```python
from build123d import *

# Parameters (mm, degrees)
PAD_DEPTH = 50
FILLET_R  = 1


with BuildPart() as part:
    # Sketch → Pad (new body)
    with BuildSketch(Plane.XZ):
        Polygon((0, 0), (0, 60), (60, 60), (60, 55), (5, 55), (5, 5), (60, 5), (80, 10), (80, 5), (60, 0), align=None)
    extrude(amount=PAD_DEPTH)

    # Fillet
    fillet_edges = [part.edges().sort_by_distance(p)[0] for p in [
        (0, -25, 0),
        (60, -25, 0),
        (80, -25, 5),
        (80, -25, 10),
        (60, -25, 55),
        (60, -25, 60),
        (0, -25, 60),
        (60, -25, 5),
        (5, -25, 5),
        (5, -25, 55),
    ]]
    fillet(fillet_edges, radius=FILLET_R)


solid = part.part
```
Check sheet for the modelled part. Datum: model origin and axes. Units: mm. A direction names the side the tool comes from. Give positions to 0.01 mm unless a question says otherwise; leave off trailing zeros. Order: outer loops, then holes, each group sorted by start corner. A loop starts at its lowest first (then second) coordinate and runs counter-clockwise, first axis right, second up. Notation, with made-up numbers: M -10,26.5 L 14,26.5 A23 ccw 14,46.5 Z; hole C 74.25,89.5 d4. An arc over 180 degrees is marked long. Answer in a Markdown table with one row per item.
1) Gauge pin test, flat ends, axial feed: P1, Ø14.5, axis at y = -31, z = 25.5, coming from the +X side; P2, Ø0.9, axis at y = -27, z = 58, coming from the +X side. Record the tip position at first contact, or that the pin passes through.
Filled sheet:
| item | result |
|---|---|
| P1 | stops at x = 5 |
| P2 | stops at x = 60 |
2) Cross-section at D-D, the plane x = 67.5. Enter the section's corners in (y, z) (3 decimals).
Filled sheet:
| item | result |
|---|---|
| outline | M -50,1.875 L 0,1.875 L 0,6.875 L -50,6.875 Z |
3) Thickness scan on L1, parallel to Z at x = 15.5, y = -10; L2, parallel to X at y = -35.5, z = 58; L3, parallel to X at y = -23, z = 24. Record the ranges inside material, lowest first. Write a range as [from, to].
Filled sheet:
| item | result |
|---|---|
| L1 | z = [0, 5], [55, 60] |
| L2 | x = [0, 60] |
| L3 | x = [0, 5] |
4) Cross-section at C-C, the plane z = 18.5. Enter the section's corners in (x, y), plus the area to 3 significant figures.
Filled sheet:
| item | result |
|---|---|
| outline | M 0,-50 L 5,-50 L 5,0 L 0,0 Z |
| area | 250 mm2 |
5) Release check for a two-part mould opening along X. For faces 1 (the flat face through (33, -25, 5)), 2 (the flat face through (4.6, 0, 25.7)), 3 (the flat face through (69.815, -24.65, 2.454)) record: +X half, -X half, draft (parallel to the pull), parting line (faces both ways), or undercut.
Filled sheet:
| item | result |
|---|---|
| face 1 | undercut |
| face 2 | draft |
| face 3 | +X half |
6) Cross-section at B-B, the plane x = 12. Enter the section's corners in (y, z).
Filled sheet:
| item | result |
|---|---|
| outline | M -50,0 L 0,0 L 0,5 L -50,5 Z; M -50,55 L 0,55 L 0,60 L -50,60 Z |
7) Cross-section at A-A, the plane y = -43.5. Enter the section's corners in (x, z).
Filled sheet:
| item | result |
|---|---|
| outline | M 0,1 A1 ccw 1,0 L 59.88,0 A1 ccw 60.12,0.03 L 79.24,4.81 A1 ccw 80,5.78 L 80,8.72 A1 ccw 78.76,9.69 L 60.12,5.03 A1 cw 59.88,5 L 6,5 A1 cw 5,6 L 5,54 A1 cw 6,55 L 59,55 A1 ccw 60,56 L 60,59 A1 ccw 59,60 L 1,60 A1 ccw 0,59 Z |
8) Access from +Z, -Z, +X, -X, +Y, -Y to the whole of each face (thin tool, end or side, straight path). Record for faces 4 (the flat face through (33, -25, 55)), 5 (the flat face through (30, -25, 60)), 6 (the flat face through (69.308, -24.65, 7.327)), 7 (the flat face through (60, -25, 58)), 8 (the flat face through (31, -25, 0)).
Filled sheet:
| item | result |
|---|---|
| face 4 | +X, +Y, -Y |
| face 5 | +Z, +X, -X, +Y, -Y |
| face 6 | +Z, +Y, -Y |
| face 7 | +Z, +X, +Y, -Y |
| face 8 | -Z, +X, -X, +Y, -Y |
